Here's the drawing with two shaded views (mm, measured from the low corner). I have some questions. Coordinates: 2 decimals unless noted, no trailing zeros. Loops run counter-clockwise (first coordinate to the right, second up) from the corner with the lowest first, then second, coordinate; pieces in that order, holes last. Notation, with made-up numbers: (-19, 48) -> (36, 48) arc R9 ccw to (36, 65) -> close; hole circle Ø3 at (56.25, 23.5). An arc over 180 degrees is marked (long way). Answer as a JSON object with one key per item and string values. Group by question number.
1) I want a section at D-D (z = 37.5). Write out the boundary of the cut face in (x, y).
2) I'm going to push a flat-ended pin straight in: pin 1 (6 mm diameter, centred on x = 88, y = 4, fed in from +Z). Where does the tip first touch, or does it pass through?
3) I want a section at A-A (x = 83.5). Write out the boundary of the cut face in (y, z).
4) I want a section at C-C (x = 60). Write out the boundary of the cut face in (y, z), then the cut area to 3 significant figures.
5) I want a section at B-B (z = 44.5). Write out the boundary of the cut face in (x, y), then the cut area to 3 significant figures.
6) I need wall thicknesses on probe 1 along Y at (x, z) = (17.5, 28.5); probe 2 along Z at (x, y) = (36, 5). Which ranges of each line are inside material? Lowest first, please. Write a range as [from, to].
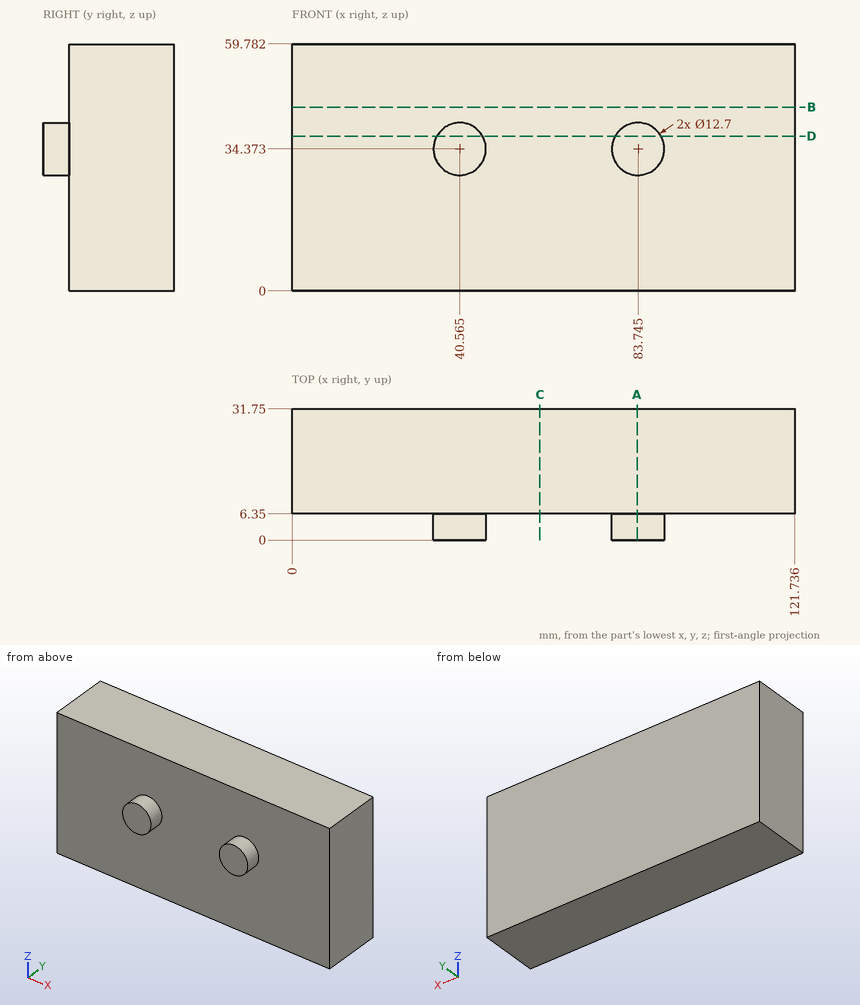
Determined:
{
 "1": {"outline": "(0, 6.35) -> (35.04, 6.35) -> (35.04, 0) -> (46.09, 0) -> (46.09, 6.35) -> (78.22, 6.35) -> (78.22, 0) -> (89.27, 0) -> (89.27, 6.35) -> (121.74, 6.35) -> (121.74, 31.75) -> (0, 31.75) -> close"},
 "2": {"pin 1": "z = 59.78"},
 "3": {"outline": "(0, 28.03) -> (6.35, 28.03) -> (6.35, 0) -> (31.75, 0) -> (31.75, 59.78) -> (6.35, 59.78) -> (6.35, 40.72) -> (0, 40.72) -> close"},
 "4": {"outline": "(6.35, 0) -> (31.75, 0) -> (31.75, 59.78) -> (6.35, 59.78) -> close", "area": "1,520 mm^2"},
 "5": {"outline": "(0, 6.35) -> (121.74, 6.35) -> (121.74, 31.75) -> (0, 31.75) -> close", "area": "3,090 mm^2"},
 "6": {"probe 1": "[6.35, 31.75]", "probe 2": "[29.96, 38.79]"}
}
